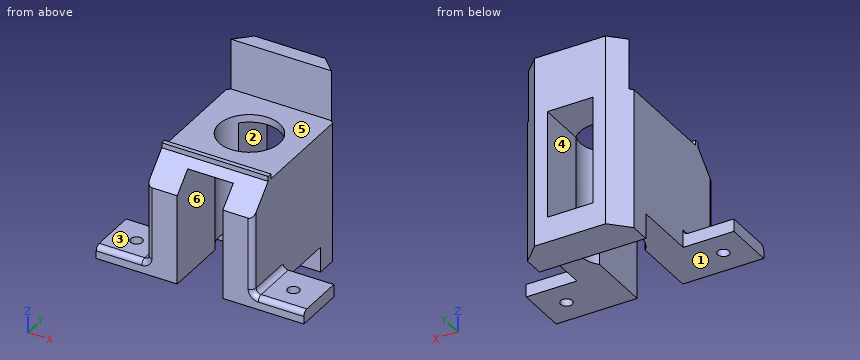
```python
from build123d import *

# Parameters (mm, degrees)
SKETCH_1_W          = 12
SKETCH_1_H          = 60
EXTRUDE_1_DEPTH     = 42.5
EXTRUDE_1_2_DEPTH   = 42.5
SKETCH_2_W          = 42
SKETCH_2_H          = 60
SKETCH_2_R          = 12
EXTRUDE_2_DEPTH     = 3
SKETCH_3_R          = 12
CUT_EXTRUDE_1_DEPTH = 79.174484328
SKETCH_4_W          = 42
SKETCH_4_H          = 15
EXTRUDE_3_DEPTH     = 10
CHAMFER_1_SIZE      = 10
SKETCH_5_W          = 5
SKETCH_5_H          = 20
EXTRUDE_4_DEPTH     = 20
HOLE_WIZARD_M4_1_D  = 4.6
FILLET_1_R          = 2
CHAMFER_2_SIZE      = 7
EXTRUDE_5_DEPTH     = 20
SKETCH_9_W          = 42
SKETCH_9_H          = 1.8
EXTRUDE_6_DEPTH     = 2


with BuildPart() as part:
    # Sketch 1 → Extrude 1 (new body)
    with BuildSketch(Plane.XY):
        with Locations((-15, 30)):
            Rectangle(SKETCH_1_W, SKETCH_1_H)
    extrude(amount=EXTRUDE_1_DEPTH)



with BuildPart() as body_2:
    # Sketch 1 → Extrude 1 2 (new body)
    with BuildSketch(Plane.XY):
        with Locations((15, 30)):
            Rectangle(SKETCH_1_W, SKETCH_1_H)
    extrude(amount=EXTRUDE_1_2_DEPTH)


with BuildPart() as part_1:
    add(part.part)

    add(body_2.part)  # Extrude 2 merges body 2
    # Sketch 2 → Extrude 2 (add)
    with BuildSketch(Plane.XY.offset(42.5)):
        with Locations((0, 30)):
            Rectangle(SKETCH_2_W, SKETCH_2_H)
        with Locations(Location((0, 33, 0), (0, 0, 138.590377891))):
            Circle(SKETCH_2_R, mode=Mode.SUBTRACT)
    extrude(amount=EXTRUDE_2_DEPTH)

    # Sketch 3 → Cut-Extrude 1 (cut, through all)
    with BuildSketch(Plane.XY.offset(45.5)):
        with Locations(Location((0, 33, 0), (0, 0, 138.590377891))):
            Circle(SKETCH_3_R)
    extrude(amount=-CUT_EXTRUDE_1_DEPTH, mode=Mode.SUBTRACT)

    # Sketch 4 → Extrude 3 (add)
    with BuildSketch(Plane(origin=(0, 0, 0), x_dir=(-1, 0, 0), z_dir=(0, 0, -1))):
        with Locations((0, 52.5)):
            Rectangle(SKETCH_4_W, SKETCH_4_H)
    extrude(amount=EXTRUDE_3_DEPTH)

    # Chamfer 1
    # the kernel refuses this chamfer: 10 mm, written as the material it takes off along each edge
    with BuildSketch(Plane(origin=(46.71682988, 0, 45.5), x_dir=(0, -0.02749587661058638, -0.9996219169112968), z_dir=(-1, 0, 0))) as chamfer_1_piece_1:
        Polygon((CHAMFER_1_SIZE * 0.999621916911, -CHAMFER_1_SIZE * 0.0274958766106), (-CHAMFER_1_SIZE * 0.0274958766106, -CHAMFER_1_SIZE * 0.999621916911), (0, 0), align=None)
    extrude(amount=93.433659759, mode=Mode.SUBTRACT)

    # Sketch 5 → Extrude 4 (add)
    with BuildSketch(Plane(origin=(21, 0, 0), x_dir=(0, 0, -1), z_dir=(1, 0, 0))):
        with Locations((-2.5, 10)):
            Rectangle(SKETCH_5_W, SKETCH_5_H)
    extrude_4 = extrude(amount=EXTRUDE_4_DEPTH)

    # Hole Wizard M4 _ _1 (through all)
    with Locations(Plane.XY.offset(5)):
        with Locations((31, 10)):
            hole_wizard_m4_1 = Hole(HOLE_WIZARD_M4_1_D / 2)

    # Mirror 1: Extrude 4, Hole Wizard M4 _ _1 across plane
    add(extrude_4.mirror(Plane(origin=(0, 0, 0), x_dir=(0, 0, 1), z_dir=(1, 0, 0))))
    add(hole_wizard_m4_1.mirror(Plane(origin=(0, 0, 0), x_dir=(0, 0, 1), z_dir=(1, 0, 0))), mode=Mode.SUBTRACT)

    # Fillet 1
    fillet_1_edges = [part_1.edges().sort_by_distance(p)[0] for p in [
        (21, 0, 20.25),
        (-21, 0, 20.25),
        (21, 10, 5),
        (31, 0, 5),
        (-31, 0, 5),
        (-21, 10, 5),
    ]]
    fillet(fillet_1_edges, radius=FILLET_1_R)

    # Chamfer 2
    chamfer_2_edges = [part_1.edges().sort_by_distance(p)[0] for p in [
        (21, 60, 17.75),
        (-21, 60, 17.75),
    ]]
    chamfer(chamfer_2_edges, length=CHAMFER_2_SIZE)

    # Sketch 8 → Extrude 5 (add)
    with BuildSketch(Plane.XY.offset(45.5)):
        Polygon((-19.8, 54.2), (19.8, 54.2), (14, 60), (-14, 60), align=None)
    extrude(amount=EXTRUDE_5_DEPTH)

    # Sketch 9 → Extrude 6 (add)
    with BuildSketch(Plane.XY.offset(45.5)):
        with Locations((0, 10.9)):
            Rectangle(SKETCH_9_W, SKETCH_9_H)
    extrude(amount=EXTRUDE_6_DEPTH)


solid = part_1.part
```
The listing builds one solid part. Answer for the finished solid, in the listing's coordinates (mm). Face numbers are marked on the shaded views. A direction names the side the tool comes from. Give positions to 0.01 mm unless a question says otherwise; leave off trailing zeros. Write each loop counter-clockwise with the first axis right and the second up, starting at its lowest first coordinate (ties: lowest second). Pieces come first, ordered by that corner, then holes. Notation, with made-up numbers: M 74.5,82.25 L 98.5,82.25 A22 cw 98.5,108.25 Z; hole C 81.5,62.5 d1. An arc over 180 degrees is marked long. Write each question's results on one line, items separated by ' | '.
Q1. Section B-B, the plane x = 31 is taken. Write down the section's boundary in (y, z).
Output values:
outline: M 0,0 L 7.7,0 L 7.7,5 L 2,5 A2 ccw 0,3 Z; M 12.3,0 L 20,0 L 20,5 L 12.3,5 Z
Q2. Section A-A, the plane y = 33 is taken. Write down the section's boundary in (x, z).
Output values:
outline: M -21,0 L -12,0 L -12,45.5 L -21,45.5 Z; M 12,0 L 21,0 L 21,45.5 L 12,45.5 Z
Q3. Flat-ended cylindrical pins translate along their axes: P1, Ø20, axis at x = -1, y = 12, coming from the -Z side; P2, Ø5.5, axis at x = -33, y = 13.5, coming from the +Z side; P3, Ø2, axis at x = -10, y = 38.5, coming from the +Z side; P4, Ø12, axis at x = 4, z = 10, coming from the -Y side. Find the tip coordinate at first contact, or state that the pin passes through.
Output values:
P1: z = 0 | P2: z = 5 | P3: z = 45.5 | P4: y = 0
Q4. A tool of negligible diameter and unlimited length cuts with its end or side. For the marked faces 1, 2 and 3, from which of +Z, -Z, +X, -X, +Y, -Y can it reach the whole face along a straight path? Write none if from no direction.
Output values:
face 1: -Z, +X, -X, -Y | face 2: +Y, -Y | face 3: +Z, -X, +Y, -Y
Q5. Section D-D, the plane y = 18 is taken. Write down the section's boundary in (x, z), then the cut area to 3 significant figures.
Output values:
outline: M -41,0 L -9,0 L -9,42.5 L 9,42.5 L 9,0 L 41,0 L 41,5 L 23,5 A2 cw 21,7 L 21,45.5 L -21,45.5 L -21,7 A2 cw -23,5 L -41,5 Z | area: 1,350 mm2
Q6. Consider L1, parallel to X at y = 10, z = 31.5; L2, parallel to X at y = 33, z = 24; L3, parallel to Z at x = -5.5, y = 48. Determine where each line is inside the solid, lowest interval first. Write a range as from..to.
Output values:
L1: -21..-9, 9..21 | L2: -21..-12, 12..21 | L3: -10..0, 42.5..45.5
Q7. Section C-C, the plane z = 28.5 is taken. Write down the section's boundary in (x, y).
Output values:
outline: M -21,2 A2 ccw -19,0 L -9,0 L -9,25.06 A12 cw -9,40.94 L -9,60 L -14,60 L -21,53 Z; M 9,0 L 19,0 A2 ccw 21,2 L 21,53 L 14,60 L 9,60 L 9,40.94 A12 cw 9,25.06 Z
Q8. For a pull along Z with two mould halves and no side action, classify the marked faces 4, 5 and 6 as released by +Z, released by -Z, zero draft, split by the parting line, or undercut.
Output values:
face 4: undercut | face 5: released by +Z | face 6: zero draft
